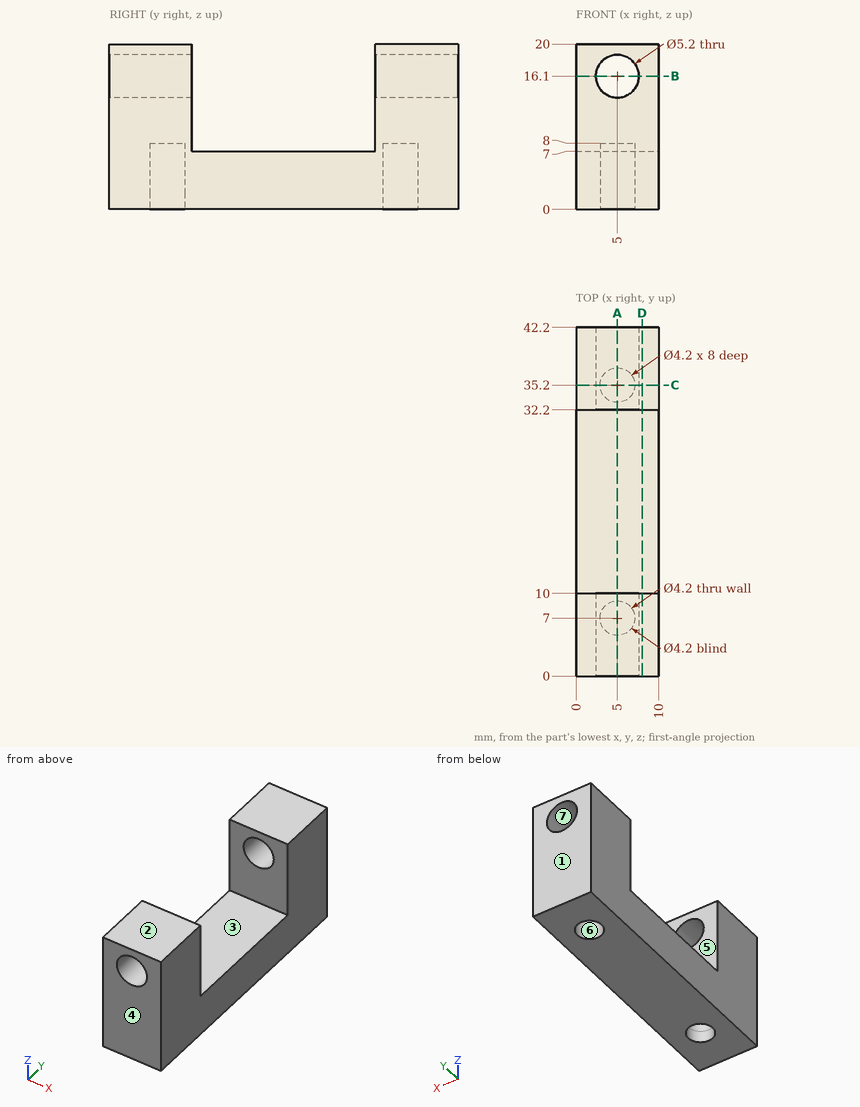
Geometry check sheet. Reference: drawing and pictorial views, mm from the part's lowest x, y, z. A direction names the side the tool comes from. Round coordinates to 2 decimals unless told otherwise and drop trailing zeros. Order: outer loops, then holes, each group sorted by start corner. A loop starts at its lowest first (then second) coordinate and runs counter-clockwise, first axis right, second up. Notation, with made-up numbers: M 20.5,2 L 46.5,2 A20 ccw 46.5,15 Z; hole C 41,46 d7. An arc over 180 degrees is marked long. One line per item, written item: value. Start each with the question number.
1. Gauge pin test, flat ends, axial feed: P1, Ø3.5, axis at x = 5, y = 7, coming from the -Z side; P2, Ø3, axis at x = 3, y = 20, coming from the +Z side. Record the tip position at first contact, or that the pin passes through.
2. Access from +Z, -Z, +X, -X, +Y, -Y to the whole of each face (thin tool, end or side, straight path). Record for the marked faces 5, 6 and 7.
3. Release check for a two-part mould opening along Y. For the marked faces 1, 2, 3 and 4 record: released by +Y, released by -Y, zero draft, split by the parting line, or undercut.
4. Section check D-D on x = 8. Enter the section's corners in (y, z).
5. Scan lines: line 1 along Y through (x, z) = (5, 2.75); line 2 along X through (y, z) = (7, 0.95); line 3 along Y through (x, z) = (0.5, 7.75). Record each from-to range of solid material in increasing order.
6. Section check B-B on z = 16.1. Enter the section's corners in (x, y), and give its area (3 significant figures).
7. Section check C-C on y = 35.2. Enter the section's corners in (x, z), and give its area (3 significant figures).
8. Section check A-A on x = 5. Enter the section's corners in (y, z), and give its area (3 significant figures).
Results found:
1. P1: z = 8
1. P2: z = 7
2. face 5: +Z, +X, -X
2. face 6: -Z
2. face 7: +Y, -Y
3. face 1: released by +Y
3. face 2: zero draft
3. face 3: undercut
3. face 4: released by -Y
4. outline: M 0,0 L 42.2,0 L 42.2,20 L 32.2,20 L 32.2,7 L 10,7 L 10,20 L 0,20 Z
5. line 1: 0 to 4.9, 9.1 to 33.1, 37.3 to 42.2
5. line 2: 0 to 2.9, 7.1 to 10
5. line 3: 0 to 10, 32.2 to 42.2
6. outline: M 0,0 L 2.4,0 L 2.4,10 L 0,10 Z; M 0,32.2 L 2.4,32.2 L 2.4,42.2 L 0,42.2 Z; M 7.6,0 L 10,0 L 10,10 L 7.6,10 Z; M 7.6,32.2 L 10,32.2 L 10,42.2 L 7.6,42.2 Z
6. area: 96.0 mm^2
7. outline: M 0,0 L 2.9,0 L 2.9,8 L 7.1,8 L 7.1,0 L 10,0 L 10,20 L 0,20 Z; hole C 5,16.1 d5.2
7. area: 145 mm^2
8. outline: M 0,0 L 4.9,0 L 4.9,8 L 9.1,8 L 9.1,0 L 33.1,0 L 33.1,8 L 37.3,8 L 37.3,0 L 42.2,0 L 42.2,13.5 L 32.2,13.5 L 32.2,7 L 10,7 L 10,13.5 L 0,13.5 Z; M 0,18.7 L 10,18.7 L 10,20 L 0,20 Z; M 32.2,18.7 L 42.2,18.7 L 42.2,20 L 32.2,20 Z
8. area: 384 mm^2
